Drawing for the job (mm, zero at the part's lowest x, y, z). A direction names the side the tool comes from. Round coordinates to 2 decimals unless told otherwise and drop trailing zeros. Write each loop counter-clockwise with the first axis right and the second up, starting at its lowest first coordinate (ties: lowest second). Pieces come first, ordered by that corner, then holes.
Item 1: Band-saw the part on D-D, the plane z = 2.2. Write the cut outline in (x, y).
Item 2: Wall check: probe 1 along Y at (x, z) = (2.5, 2.2); probe 2 along Y at (x, z) = (2.5, 1.3) (3 decimals); probe 3 along Z at (x, y) = (1, 0.7). Give the ranges that are in metal, low to high.
Item 3: Band-saw the part on A-A, the plane y = 2.5. Write the cut outline in (x, z) (3 decimals), then the cut area to 3 significant figures.
Item 4: Band-saw the part on C-C, the plane z = 3.35. Write the cut outline in (x, y), then the cut area to 3 significant figures.
Item 5: Mould opens along X. For the marked faces 3, 4 and 5 say: +X half, -X half, draft (parallel to the pull), parting line (faces both ways), or undercut.
Item 6: 3-axis set-ups, long thin cutter, end or side, ignore diameter. For the marked faces 1 and 2: which of +Z, -Z, +X, -X, +Y, -Y reach the whole face in a straight line?
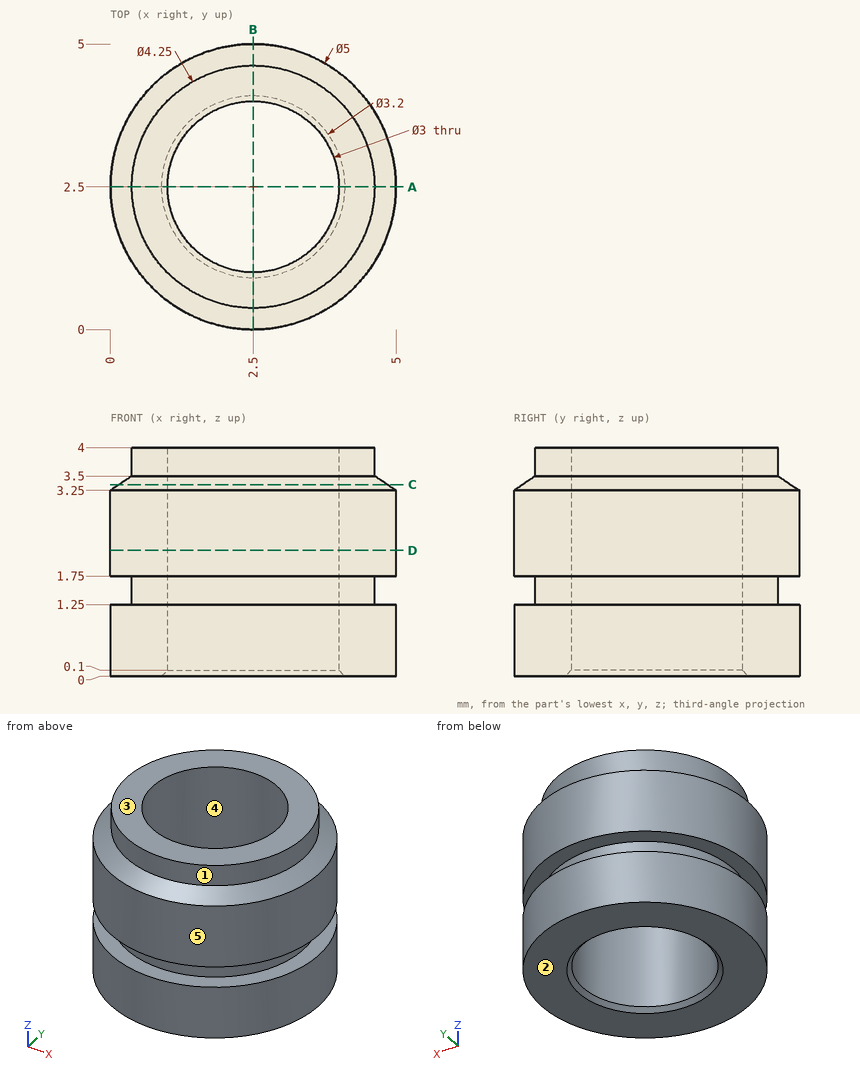
Results:
1. outline: circle Ø5 at (2.5, 2.5); hole circle Ø3 at (2.5, 2.5)
2. probe 1: y = 0 to 1, 4 to 5
2. probe 2: y = 0.375 to 1, 4 to 4.625
2. probe 3: z = 0 to 1.25, 1.75 to 3.35
3. outline: (0, 0) - (0.9, 0) - (1, 0.1) - (1, 4) - (0.375, 4) - (0.375, 3.5) - (0, 3.25) - (0, 1.75) - (0.375, 1.75) - (0.375, 1.25) - (0, 1.25) - close; (4, 0.1) - (4.1, 0) - (5, 0) - (5, 1.25) - (4.625, 1.25) - (4.625, 1.75) - (5, 1.75) - (5, 3.25) - (4.625, 3.5) - (4.625, 4) - (4, 4) - close
3. area: 7.15 mm2
4. outline: circle Ø4.7 at (2.5, 2.5); hole circle Ø3 at (2.5, 2.5)
4. area: 10.3 mm2
5. face 3: draft
5. face 4: undercut
5. face 5: parting line
6. face 1: +Z
6. face 2: -Z, +X, -X, +Y, -Y
